Check sheet for the modelled part. Datum: model origin and axes. Units: mm. A direction names the side the tool comes from. Give positions to 0.01 mm unless a question says otherwise; leave off trailing zeros. Order: outer loops, then holes, each group sorted by start corner. A loop starts at its lowest first (then second) coordinate and runs counter-clockwise, first axis right, second up. Notation, with made-up numbers: (75, -22.75) -> (92, -22.75) arc R10 cw to (92, -10.75) -> close; hole circle Ø8 at (87, -15.75). An arc over 180 degrees is marked (long way). Write each question's results on one line, items separated by ' | '.
from build123d import *

# Parameters (mm, degrees)
SKETCH1_R           = 24.255
BOSS_EXTRUDE1_DEPTH = 15
SKETCH2_R           = 12
BOSS_EXTRUDE2_DEPTH = 10
SKETCH3_R           = 5
CUT_EXTRUDE1_DEPTH  = 26
SKETCH4_R           = 24.255
SKETCH4_R_2         = 15.915
CUT_EXTRUDE3_DEPTH  = 15
SKETCH5_R           = 17.5
SKETCH5_R_2         = 15.915
BOSS_EXTRUDE3_DEPTH = 1.5
SKETCH6_R           = 17.5
SKETCH6_R_2         = 15.915
BOSS_EXTRUDE4_DEPTH = 1.5
SCALE1_SCALE        = 1.5


with BuildPart() as part:
    # Sketch1 → Boss-Extrude1 (new body)
    with BuildSketch(Plane(origin=(0, 0, 0), x_dir=(1, 0, 0), z_dir=(0, 1, 0))):
        Circle(SKETCH1_R)
    extrude(amount=BOSS_EXTRUDE1_DEPTH)

    # Sketch2 → Boss-Extrude2 (add)
    with BuildSketch(Plane(origin=(0, 15, 0), x_dir=(1, 0, 0), z_dir=(0, 1, 0))):
        Circle(SKETCH2_R)
    extrude(amount=BOSS_EXTRUDE2_DEPTH)

    # Sketch3 → Cut-Extrude1 (cut)
    with BuildSketch(Plane(origin=(0, 25, 0), x_dir=(1, 0, 0), z_dir=(0, 1, 0))):
        Circle(SKETCH3_R)
    extrude(amount=-CUT_EXTRUDE1_DEPTH, mode=Mode.SUBTRACT)

    # Sketch4 → Cut-Extrude3 (cut)
    with BuildSketch(Plane.XZ):
        Circle(SKETCH4_R)
        Circle(SKETCH4_R_2, mode=Mode.SUBTRACT)
    extrude(amount=-CUT_EXTRUDE3_DEPTH, mode=Mode.SUBTRACT)

    # Sketch5 → Boss-Extrude3 (add)
    with BuildSketch(Plane.XZ):
        Circle(SKETCH5_R)
        Circle(SKETCH5_R_2, mode=Mode.SUBTRACT)
    extrude(amount=-BOSS_EXTRUDE3_DEPTH)

    # Sketch6 → Boss-Extrude4 (add)
    with BuildSketch(Plane(origin=(0, 15, 0), x_dir=(1, 0, 0), z_dir=(0, 1, 0))):
        Circle(SKETCH6_R)
        Circle(SKETCH6_R_2, mode=Mode.SUBTRACT)
    extrude(amount=-BOSS_EXTRUDE4_DEPTH)


with BuildPart() as part_1:
    # Scale1: scaled about (0, 10.616360153, 0)
    add(part.part.scale(SCALE1_SCALE).moved(Location((0, -5.308180077, 0))))


solid = part_1.part
1. Section check A-A on z = 0. Record the cut outline in (x, y), then the cut area to 3 significant figures.
Verdict:
outline: (-26.25, -5.31) -> (-7.5, -5.31) -> (-7.5, 32.19) -> (-18, 32.19) -> (-18, 17.19) -> (-26.25, 17.19) -> (-26.25, 14.94) -> (-23.87, 14.94) -> (-23.87, -3.06) -> (-26.25, -3.06) -> close; (7.5, -5.31) -> (26.25, -5.31) -> (26.25, -3.06) -> (23.87, -3.06) -> (23.87, 14.94) -> (26.25, 14.94) -> (26.25, 17.19) -> (18, 17.19) -> (18, 32.19) -> (7.5, 32.19) -> close | area: 1,070 mm^2
2. Mould release check, pull along Z, two halves, no side actions. Record for faces 4 (the cylindrical face through (-7.493, 13.704, -0.33)), 5 (the flat face through (5.5, -5.308, -5.5)), 6 (the cylindrical face through (-2.343, 24.587, -17.847)): +Z half, -Z half, draft (parallel to the pull), parting line (faces both ways), or undercut.
Verdict:
face 4: undercut | face 5: draft | face 6: parting line
3. Access from +Z, -Z, +X, -X, +Y, -Y to the whole of each face (thin tool, end or side, straight path). Record for faces 1 (the flat face through (12, 14.942, 21)), 2 (the flat face through (-6.2, 17.192, 17.1)), 3 (the cylindrical face through (25, 16, -8)).
Verdict:
face 1: none | face 2: +Y | face 3: +Y, -Y
4. Gauge pin test, flat ends, axial feed: pin 1 Ø8 at (x, y) = (19, 17) entering from +Z; pin 2 Ø1 at (x, y) = (-16, 1.5) entering from -Z; pin 3 Ø6 at (x, y) = (17, 2) entering from -Z. Record the tip position at first contact, or that the pin passes through.
Verdict:
pin 1: stops at z = 21.54 | pin 2: stops at z = -18.16 | pin 3: stops at z = -19.34
5. Section check C-C on y = 6. Record the cut outline in (x, z) (1 decimal).
Verdict:
outline: circle Ø47.7 at (0, 0); hole circle Ø15 at (0, 0)
6. Section check B-B on x = 0. Record the cut outline in (y, z), then the cut area to 3 significant figures.
Verdict:
outline: (-5.31, -26.25) -> (-3.06, -26.25) -> (-3.06, -23.87) -> (14.94, -23.87) -> (14.94, -26.25) -> (17.19, -26.25) -> (17.19, -18) -> (32.19, -18) -> (32.19, -7.5) -> (-5.31, -7.5) -> close; (-5.31, 7.5) -> (32.19, 7.5) -> (32.19, 18) -> (17.19, 18) -> (17.19, 26.25) -> (14.94, 26.25) -> (14.94, 23.87) -> (-3.06, 23.87) -> (-3.06, 26.25) -> (-5.31, 26.25) -> close | area: 1,070 mm^2
7. Material ranges on probe 1 along Z at (x, y) = (0, 23); probe 2 along X at (y, z) = (3, 0); probe 3 along X at (y, z) = (16.5, 0), recorded low to high. Write a range as from..to.
Verdict:
probe 1: z = -18..-7.5, 7.5..18 | probe 2: x = -23.87..-7.5, 7.5..23.87 | probe 3: x = -26.25..-7.5, 7.5..26.25
8. Section check D-D on x = -19.5. Record the cut outline in (y, z), then the cut area to 3 significant figures.
Verdict:
outline: (-5.31, -17.57) -> (-3.06, -17.57) -> (-3.06, -13.77) -> (14.94, -13.77) -> (14.94, -17.57) -> (17.19, -17.57) -> (17.19, 17.57) -> (14.94, 17.57) -> (14.94, 13.77) -> (-3.06, 13.77) -> (-3.06, 17.57) -> (-5.31, 17.57) -> close | area: 654 mm^2
